Geometry: final body of the model. Coordinates: model frame, mm. A direction names the side the tool comes from. Round coordinates to 2 decimals unless told otherwise and drop trailing zeros. Loops run counter-clockwise (first coordinate to the right, second up) from the corner with the lowest first, then second, coordinate; pieces in that order, holes last. Notation, with made-up numbers: (44.25, 71) - (96.25, 71) arc R17 ccw to (96.25, 83) - close; hole circle Ø9 at (82.5, 84). An arc over 180 degrees is marked (long way). Use CSV: the item, a comma, the result in double quotes.
Solid Edge part; units mm, degrees
sketch "Sketch1" plane through (0, 0, 0) normal (0, 0, 1) x (1, 0, 0)
  line L0 (30, 22.5) -> (-30, 22.5)
  line L1 (-30, 22.5) -> (-30, -22.5)
  line L2 (-30, -22.5) -> (30, -22.5)
  line L3 (30, -22.5) -> (30, 22.5)
extrude "Protrusion1" add sketch "Sketch1" along normal blind 40
sketch "Sketch2" plane through (0, -22.5, 12.5) normal (0, -1, 0) x (1, 0, 0)
  line L0 (7.5, 0.5) -> (-7.5, 0.5)
  line L1 (-7.5, 0.5) -> (-7.5, -9.5)
  line L2 (-7.5, -9.5) -> (7.5, -9.5)
  line L3 (7.5, -9.5) -> (7.5, 0.5)
  dimension "D1" = 7.5
  dimension "D2" = 7.5
extrude "ExtrudedCutout_1" cut sketch "Sketch2" against normal blind 70.2135
fillet "Verrundung_2" radius 4 4 edges at (7.5, 0, 13) (-7.5, 0, 13) (-7.5, 0, 3) (7.5, 0, 3)
sketch "Sketch3" plane through (0, 0, 40) normal (0, 0, 1) x (1, 0, 0)
  circle A0 centre (-18, 0) radius 6
extrude "ExtrudedCutout_3" cut sketch "Sketch3" against normal blind 20.7766
fillet "Round_3" radius 1 12 edges at (0, -22.5, 40) (-30, 0, 40) (-30, -22.5, 20) (30, -22.5, 20) (30, 0, 40) (0, 22.5, 40) (-30, 22.5, 20) (0, 22.5, 0) (-30, 0, 0) (0, -22.5, 0) (30, 0, 0) (30, 22.5, 20)
sketch "Sketch4" plane through (0, 0, 40) normal (0, 0, 1) x (1, 0, 0)
  line L0 (-27.5, -20) -> (27.5, -20)
  line L1 (27.5, -20) -> (27.5, 20)
  line L2 (27.5, 20) -> (-27.5, 20)
  line L3 (-27.5, 20) -> (-27.5, -20)
extrude "ExtrudedCutout_5" cut sketch "Sketch4" against normal blind 38
hole "Hole1" at (0, 12.5, 21) direction (0, 0, -1) diameter 3.4 end up to next
hole "Hole2" at (0, -12.5, 21) direction (0, 0, -1) diameter 3.4 end up to next
sketch "Sketch5" plane through (0, 0, 2) normal (0, 0, 1) x (1, 0, 0)
  circle A0 centre (-5, 7) radius 1.6
  circle A1 centre (-5, 7) radius 2.9
  circle A2 centre (-5, -7) radius 1.6
  circle A3 centre (-5, -7) radius 2.9
extrude "Protrusion2" add sketch "Sketch5" along normal blind 8
Item 1: Reachability of faces 1 (the flat face through (-5, 7, 2)), 2 (the cylindrical face through (-6.297, -21.232, 4.141)), 3 (the flat face through (0, 21, 13)) from +Z, -Z, +X, -X, +Y, -Y: full face, straight path, thin tool, end or side. Return the list, or none.
Final values:
face 1,"+Z"
face 2,"-Y"
face 3,"+Y, -Y"
Item 2: Section D-D on x = -11. Return the cut outline in (y, z).
Final values:
outline,"(-22.5, 1) arc R1 ccw to (-21.5, 0) - (21.5, 0) arc R1 ccw to (22.5, 1) - (22.5, 39) arc R1 ccw to (21.5, 40) - (20, 40) - (20, 2) - (-20, 2) - (-20, 40) - (-21.5, 40) arc R1 ccw to (-22.5, 39) - close"
Item 3: Pin query (flat end, axial travel): P1, Ø3.5, axis at x = -4.5, y = -7, coming from the +Z side; P2, Ø5, axis at x = 21, y = -2, coming from the +Z side. Return the tip coordinate at first contact, or that it passes through.
Final values:
P1,"stops at z = 10"
P2,"stops at z = 2"
Item 4: Mould query, pull axis Z, two halves, no side actions, for faces 4 (the cylindrical face through (0.51, -14.12, 1.01)), 5 (the flat face through (0, 0, 2)), 6 (the flat face through (-7.5, -21, 8)). Classes: released by +Z, released by -Z, zero draft, split by the parting line, or undercut.
Final values:
face 4,"zero draft"
face 5,"released by +Z"
face 6,"undercut"
Item 5: Section A-A on x = 0. Return the cut outline in (y, z).
Final values:
outline,"(-22.5, 1) arc R1 ccw to (-21.5, 0) - (-14.2, 0) - (-14.2, 2) - (-20, 2) - (-20, 3) - (-22.5, 3) - close; (-22.5, 13) - (-20, 13) - (-20, 40) - (-21.5, 40) arc R1 ccw to (-22.5, 39) - close; (-10.8, 0) - (10.8, 0) - (10.8, 2) - (-10.8, 2) - close; (14.2, 0) - (21.5, 0) arc R1 ccw to (22.5, 1) - (22.5, 3) - (20, 3) - (20, 2) - (14.2, 2) - close; (20, 13) - (22.5, 13) - (22.5, 39) arc R1 ccw to (21.5, 40) - (20, 40) - close"
Item 6: Section B-B on z = 19. Return the cut outline in (x, y), plus the area to 3 significant figures.
Final values:
outline,"(-30, -21.5) arc R1 ccw to (-29, -22.5) - (29, -22.5) arc R1 ccw to (30, -21.5) - (30, 21.5) arc R1 ccw to (29, 22.5) - (-29, 22.5) arc R1 ccw to (-30, 21.5) - close; hole (-27.5, -20) - (27.5, -20) - (27.5, 20) - (-27.5, 20) - close"
area,"499 mm²"
Item 7: Section C-C on y = 18. Return the cut outline in (x, z), plus the area to 3 significant figures.
Final values:
outline,"(-30, 1) arc R1 ccw to (-29, 0) - (29, 0) arc R1 ccw to (30, 1) - (30, 39) arc R1 ccw to (29, 40) - (27.5, 40) - (27.5, 2) - (-27.5, 2) - (-27.5, 40) - (-29, 40) arc R1 ccw to (-30, 39) - close"
area,"309 mm²"
Item 8: Material intervals for line 1 (Y direction, x = -5, z = 6.25); line 2 (Y direction, x = -15, z = 6); line 3 (X direction, y = -6.5, z = 34.5), sorted ascending.
Final values:
line 1,"y = -9.9 to -8.6, -5.4 to -4.1, 4.1 to 5.4, 8.6 to 9.9"
line 2,"y = -22.5 to -20, 20 to 22.5"
line 3,"x = -30 to -27.5, 27.5 to 30"
